from build123d import *

# Parameters (mm, degrees)
F2_S5_R     = 6.5
F2_T6_DEPTH = 13
F4_DEPTH    = 10
F5_R        = 1.65
F6_DEPTH    = 8.301


# Not quite as in the source:
# - a fillet or chamfer that OpenCascade refuses, or shapes differently, is made with other operations: its cross-section is extruded or revolved along the edge and cut away or added


with BuildPart() as f1:
    # F0 (on Front) → F1 (revolve)
    with BuildSketch(Plane.XZ):
        Polygon((0, 6.5), (0, 4.95), (9.6, 4.95), (10, 4.55), (11, 4.55), (11, 5.25), (38, 7.3), (38, 8.3), (9, 8.3), (9, 6.5), align=None)
    revolve(axis=Axis((19, 0, 0), (1, 0, 0)))

    # F2: chamfer of 1.9 on 1 edges, made by hand


with BuildPart() as f2_tool2:
    # F2_s3 → F2_t4 (revolve)
    with BuildSketch(Plane.XZ):
        Polygon((10.9, 8.3), (9, 6.4), (9, 8.3), align=None)
    revolve(axis=Axis((9, 0, 0), (1, 0, 0)))

    # F2_s5 → F2_t6 (cut, symmetric)
    with BuildSketch(Plane.YZ.offset(9.9)):
        Circle(F2_S5_R)
    extrude(amount=F2_T6_DEPTH, both=True, mode=Mode.SUBTRACT)


with BuildPart() as f1_1:
    add(f1.part)

    # F2_t1: cut F2_tool2
    add(f2_tool2.part, mode=Mode.SUBTRACT)

    # F3 (on face) → F4 (cut)
    with BuildSketch(Plane.YZ.offset(11)):
        with BuildLine():
            Line((-4.6153846154, 2.502144051), (-4, 2.1685248442))
            ThreePointArc((-4, 2.1685248442), (0, 4.55), (4, 2.1685248442))
            Line((4, 2.1685248442), (4.6153846154, 2.502144051))
            ThreePointArc((4.6153846154, 2.502144051), (0, 5.25), (-4.6153846154, 2.502144051))
        make_face()
    extrude(amount=-F4_DEPTH, mode=Mode.SUBTRACT)

    # F5 (on Front) → F6 (cut, through all)
    with BuildSketch(Plane.XZ):
        with Locations((29.9, 0)):
            Circle(F5_R)
    extrude(amount=F6_DEPTH, mode=Mode.SUBTRACT)


solid = f1_1.part
Check sheet for the modelled part. Datum: model origin and axes. Units: mm. A direction names the side the tool comes from. Round coordinates to 2 decimals unless told otherwise and drop trailing zeros. Order: outer loops, then holes, each group sorted by start corner. A loop starts at its lowest first (then second) coordinate and runs counter-clockwise, first axis right, second up. Notation, with made-up numbers: M 79.25,-31.75 L 111.25,-31.75 A34 ccw 111.25,5.25 Z; hole C 14,-2.5 d1. An arc over 180 degrees is marked long. One line per item, written item: value. Start each with the question number.
1. Scan lines: line 1 along Y through (x, z) = (7.25, 0); line 2 along Y through (x, z) = (5.5, 3.75); line 3 along X through (y, z) = (5, 1). Record each from-to range of solid material in increasing order.
2. Section check A-A on y = 0. Enter the section's corners in (x, z), and give its area (3 significant figures).
3. Section check C-C on x = 6. Enter the section's corners in (y, z), and give its area (3 significant figures).
4. Section check D-D on x = 29.9. Enter the section's corners in (y, z) (3 decimals), and give its area (3 significant figures).
5. Section check B-B on z = 0. Enter the section's corners in (x, y).
6. Gauge pin test, flat ends, axial feed: P1, Ø8, axis at x = 30.5, y = -1.5, coming from the +Z side; P2, Ø6, axis at y = 1, z = -0.5, coming from the +X side; P3, Ø1, axis at x = 34, z = -1.5, coming from the -Y side; P4, Ø1.5, axis at x = 9, z = 5.5, coming from the +Y side. Record the tip position at first contact, or that the pin passes through.
7. Access from +Z, -Z, +X, -X, +Y, -Y to the whole of each face (thin tool, end or side, straight path). Record for faces 4 (the cylindrical face through (28.25, -7.37, 0.07)), 5 (the cylindrical face through (10.51, -0.13, -4.55)), 6 (the flat face through (11, 1, -5)), 7 (the cylindrical face through (4.867, -0.218, -4.945)), 8 (the flat face through (0, 5, 2)).
8. Release check for a two-part mould opening along Z. For faces 1 (the flat face through (38, 7, -3)), 2 (the cylindrical face through (24.26, 8.103, -1.799)), 3 (the conical face through (9.89, -0.13, -4.66)) record: released by +Z, released by -Z, zero draft, split by the parting line, or undercut.
Results found:
1. line 1: -6.5 to -4.95, 4.95 to 6.5
1. line 2: -5.31 to -3.67, 3.67 to 5.31
1. line 3: 0 to 11
2. outline: M 0,-6.5 L 9.1,-6.5 L 10.9,-8.3 L 38,-8.3 L 38,-7.3 L 11,-5.25 L 11,-4.55 L 10,-4.55 L 9.6,-4.95 L 0,-4.95 Z; M 0,4.95 L 1,4.95 L 1,5.25 L 11,5.25 L 38,7.3 L 38,8.3 L 10.9,8.3 L 9.1,6.5 L 0,6.5 Z
2. area: 145 mm^2
3. outline: C 0,0 d13; hole M -4.62,2.5 L -4.35,2.36 A4.95 ccw long 4.35,2.36 L 4.62,2.5 A5.25 ccw Z
3. area: 52.5 mm^2
4. outline: M -8.134,-1.65 A8.3 ccw long -8.134,1.65 L -6.478,1.65 A6.685 cw long -6.478,-1.65 Z
4. area: 70.7 mm^2
5. outline: M 0,-6.5 L 9.1,-6.5 L 10.9,-8.3 L 28.25,-8.3 L 28.25,-6.56 L 11,-5.25 L 11,-4.55 L 10,-4.55 L 9.6,-4.95 L 0,-4.95 Z; M 0,4.95 L 9.6,4.95 L 10,4.55 L 11,4.55 L 11,5.25 L 38,7.3 L 38,8.3 L 10.9,8.3 L 9.1,6.5 L 0,6.5 Z; M 31.55,-8.3 L 38,-8.3 L 38,-7.3 L 31.55,-6.81 Z
6. P1: z = 8.3
6. P2: through
6. P3: y = -8.24
6. P4: y = 4.85
7. face 4: -Y
7. face 5: +X, -X
7. face 6: +X
7. face 7: -X
7. face 8: +Z, -Z, -X, +Y, -Y
8. face 1: zero draft
8. face 2: split by the parting line
8. face 3: undercut
